Work out the finished part from the listing and answer in its coordinate system (mm). Face numbers are marked on the shaded views. A direction names the side the tool comes from. Round coordinates to 2 decimals unless told otherwise and drop trailing zeros. Loops run counter-clockwise (first coordinate to the right, second up) from the corner with the lowest first, then second, coordinate; pieces in that order, holes last. Notation, with made-up numbers: (-29, 50.25) - (-18, 50.25) arc R23 cw to (-18, 79.25) - close; hole circle Ø7 at (-3, 82.5). An arc over 180 degrees is marked (long way). Return JSON: item names as keys, results as strings.
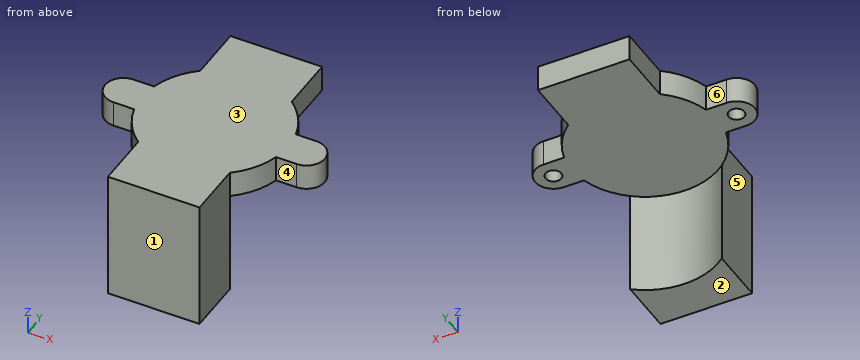
Autodesk Fusion 360 part; units mm, degrees
sketch "Sketch1" plane through (0, 0, 24.0553) normal (0, 0, 1) x (-1, 0, 0)
  line L0 (10.7499, 16.3506) -> (10.7499, 5.6583)
  line L1 (10.7499, 5.6583) -> (-6.7501, 5.6583)
  line L2 (-6.7501, 5.6583) -> (-6.7501, 16.3506)
  arc A0 (-11.5555, 23.7794) -> (-6.7501, 16.3506) centre (1.9999, 27.2794) ccw
  line L3 (-11.5555, 23.7794) -> (-15.5001, 23.7794)
  arc A1 (-15.5001, 30.7794) -> (-15.5001, 23.7794) centre (-15.5001, 27.2794) ccw
  line L4 (-15.5001, 30.7794) -> (-11.5555, 30.7794)
  arc A2 (-6.7501, 38.2081) -> (-11.5555, 30.7794) centre (1.9999, 27.2794) ccw
  line L5 (-6.7501, 38.2081) -> (-6.7501, 48.9005)
  line L6 (-6.7501, 48.9005) -> (10.7499, 48.9005)
  line L7 (10.7499, 48.9005) -> (10.7499, 38.2081)
  arc A3 (15.5554, 30.7794) -> (10.7499, 38.2081) centre (1.9999, 27.2794) ccw
  line L8 (15.5554, 30.7794) -> (19.4999, 30.7794)
  arc A4 (19.4999, 23.7794) -> (19.4999, 30.7794) centre (19.4999, 27.2794) ccw
  line L9 (19.4999, 23.7794) -> (15.5554, 23.7794)
  arc A5 (10.7499, 16.3506) -> (15.5554, 23.7794) centre (1.9999, 27.2794) ccw
  arc A6 (51.4999, 44.5294) -> (41.4999, 54.5294) centre (41.4999, 44.5294) ccw
  line L10 (41.4999, 54.5294) -> (-37.5001, 54.5294)
  arc A7 (-37.5001, 54.5294) -> (-47.5001, 44.5294) centre (-37.5001, 44.5294) ccw
  line L11 (-47.5001, 44.5294) -> (-47.5001, -34.4706)
  arc A8 (-47.5001, -34.4706) -> (-37.5001, -44.4706) centre (-37.5001, -34.4706) ccw
  line L12 (-37.5001, -44.4706) -> (41.4999, -44.4706)
  arc A9 (41.4999, -44.4706) -> (51.4999, -34.4706) centre (41.4999, -34.4706) ccw
  line L13 (51.4999, -34.4706) -> (51.4999, 44.5294)
  line L14 (42.9999, -37.9706) -> (-39.0001, -37.9706)
  line L15 (-39.0001, -37.9706) -> (-39.0001, 0.0294)
  line L16 (-39.0001, 0.0294) -> (42.9999, 0.0294)
  line L17 (42.9999, 0.0294) -> (42.9999, -37.9706)
  line L18 (10.7499, 48.9005) -> (10.7499, 38.2081)
  line L19 (-6.7501, 48.9005) -> (10.7499, 48.9005)
  line L20 (-6.7501, 38.2081) -> (-6.7501, 48.9005)
  arc A10 (-6.7501, 38.2081) -> (-11.5555, 30.7794) centre (1.9999, 27.2794) ccw
  arc A11 (15.5554, 30.7794) -> (10.7499, 38.2081) centre (1.9999, 27.2794) ccw
  line L21 (15.5554, 30.7794) -> (19.4999, 30.7794)
  arc A12 (19.4999, 23.7794) -> (19.4999, 30.7794) centre (19.4999, 27.2794) ccw
  line L22 (19.4999, 23.7794) -> (15.5554, 23.7794)
  arc A13 (15.5524, 23.7794) -> (15.5583, 30.7794) centre (1.9999, 27.2908) ccw
  line L23 (15.5524, 23.7794) -> (19.4999, 23.7794)
  arc A14 (19.4999, 23.7794) -> (19.4999, 30.7794) centre (19.4999, 27.2794) ccw
  line L24 (19.4999, 30.7794) -> (15.5583, 30.7794)
  circle A15 centre (19.4999, 27.2794) radius 2
  arc A16 (-11.5585, 30.7794) -> (-11.5526, 23.7794) centre (1.9999, 27.2908) ccw
  line L25 (-11.5585, 30.7794) -> (-15.5001, 30.7794)
  arc A17 (-15.5001, 30.7794) -> (-15.5001, 23.7794) centre (-15.5001, 27.2794) ccw
  line L26 (-15.5001, 23.7794) -> (-11.5526, 23.7794)
  circle A18 centre (-15.5001, 27.2794) radius 2
  line L27 (-6.7501, 5.6583) -> (-6.7501, 16.3506)
  line L28 (10.7499, 5.6583) -> (-6.7501, 5.6583)
  line L29 (10.7499, 16.3506) -> (10.7499, 5.6583)
  circle A19 centre (1.9999, 27.2908) radius 14
  arc A20 (-15.5001, 30.7794) -> (-15.5001, 23.7794) centre (-15.5001, 27.2794) ccw
  line L30 (-15.5001, 30.7794) -> (-11.5555, 30.7794)
  line L31 (-11.5555, 23.7794) -> (-15.5001, 23.7794)
  arc A21 (-11.5555, 23.7794) -> (-6.7501, 16.3506) centre (1.9999, 27.2794) ccw
  arc A22 (10.7499, 16.3506) -> (15.5554, 23.7794) centre (1.9999, 27.2794) ccw
  circle A23 centre (1.9999, 27.2908) radius 13
  circle A24 centre (19.4999, 27.2794) radius 1.5
  circle A25 centre (-15.5001, 27.2794) radius 1.5
extrude "Extrude2" add sketch "Sketch1" against normal blind 5 contours L0 L1 L2 A0 A5 L23 L26 L27 L28 L29 A19 A21 A22 | L8 A4 L9 L21 A12 L22 A13 L23 A14 L24 A19 | L4 A2 L5 L7 A3 L8 L18 L20 A10 A11 L21 A13 A16 A19 L30 | L3 A1 L4 A16 L25 A17 L26 A19 A20 L30 L31 | L7 A3 L8 L18 A11 L21 A19 | L4 A2 L5 L20 A10 A19 L30 | A23 makes body 1
extrude "Extrude1" add sketch "Sketch1" against normal blind 25 separate body contours L5 L6 L7 L18 L19 L20 A19 makes body 2
extrude "Extrude3" add sketch "Sketch1" against normal blind 4 separate body contours A15 | A18 makes body 3 at (-21.4974, -27.1797, 21.3887) makes body 4 at (13.5026, -27.1797, 21.3887)
sketch "Sketch2" plane through (0, 0, 24.0553) normal (0, 0, 1) x (-1, 0, 0)
  circle A0 centre (19.4999, 27.2794) radius 1.5
  circle A1 centre (19.4999, 27.2794) radius 1.5
extrude "Extrude4" add sketch "Sketch2" against normal blind 2 bodies 3
sketch "Sketch3" plane through (0, 0, 24.0553) normal (0, 0, 1) x (-1, 0, 0)
  circle A0 centre (-15.5001, 27.2794) radius 1.5
  circle A1 centre (-15.5001, 27.2794) radius 1.5
extrude "Extrude5" add sketch "Sketch3" against normal blind 2 bodies 4
extrude "Extrude6" add 1 faces at (13.7846, -26.6463, 20.0553) along direction (0, 0, -1) blind 1 on bodies 4 bodies 4 1
extrude "Extrude7" add 1 faces at (-18.7404, -28.9428, 20.0553) along direction (0, 0, -1) blind 1 on bodies 3 bodies 3 2 4
sketch "Sketch4" plane through (0, 0, 24.0553) normal (0, 0, 1) x (-1, 0, 0)
  line L0 (10.7499, 5.6583) -> (10.7499, 16.3506)
  arc A0 (10.7499, 16.3506) -> (15.5554, 23.7794) centre (1.9999, 27.2794) ccw
  line L1 (15.5554, 23.7794) -> (19.4999, 23.7794)
  arc A1 (19.4999, 23.7794) -> (19.4999, 30.7794) centre (19.4999, 27.2794) ccw
  line L2 (19.4999, 30.7794) -> (15.5554, 30.7794)
  arc A2 (15.5554, 30.7794) -> (10.7499, 38.2081) centre (1.9999, 27.2794) ccw
  line L3 (10.7499, 38.2081) -> (10.7499, 38.2196)
  arc A3 (10.7499, 38.2196) -> (-6.7501, 38.2196) centre (1.9999, 27.2908) ccw
  line L4 (-6.7501, 38.2196) -> (-6.7501, 38.2081)
  arc A4 (-6.7501, 38.2081) -> (-11.5555, 30.7794) centre (1.9999, 27.2794) ccw
  line L5 (-11.5555, 30.7794) -> (-15.5001, 30.7794)
  arc A5 (-15.5001, 30.7794) -> (-15.5001, 23.7794) centre (-15.5001, 27.2794) ccw
  line L6 (-15.5001, 23.7794) -> (-11.5555, 23.7794)
  arc A6 (-11.5555, 23.7794) -> (-6.7501, 16.3506) centre (1.9999, 27.2794) ccw
  line L7 (-6.7501, 16.3506) -> (-6.7501, 5.6583)
  line L8 (-6.7501, 5.6583) -> (10.7499, 5.6583)
  line L9 (10.7499, 48.9005) -> (-6.7501, 48.9005)
  line L10 (-6.7501, 48.9005) -> (-6.7501, 38.2196)
  arc A7 (10.7499, 38.2196) -> (-6.7501, 38.2196) centre (1.9999, 27.2908) ccw
  line L11 (10.7499, 38.2196) -> (10.7499, 48.9005)
  line L12 (10.7499, 38.2196) -> (10.7499, 48.9005)
  line L13 (-6.7501, 48.9005) -> (-6.7501, 38.2196)
  circle A8 centre (1.9999, 27.2908) radius 14
extrude "Extrude8" add sketch "Sketch4" against normal blind 25 contours A3 L9 L10 A7 L11 L12 L13 A8 bodies 2 3
1) Section A-A (z = 21) is taken. Give the vertices of the cut face in (x, y), and give its area (3 significant figures).
Verdict:
{"outline": "(-19.5, -30.78) - (-15.56, -30.78) arc R14 ccw to (-10.75, -38.22) - (-10.75, -48.9) - (6.75, -48.9) - (6.75, -38.22) arc R14 ccw to (11.56, -30.78) - (15.5, -30.78) arc R3.5 ccw to (15.5, -23.78) - (11.56, -23.78) arc R14 ccw to (6.75, -16.35) - (6.75, -5.66) - (-10.75, -5.66) - (-10.75, -16.35) arc R14 ccw to (-15.56, -23.78) - (-19.5, -23.78) arc R3.5 ccw to start; hole circle Ø3 at (-19.5, -27.28); hole circle Ø3 at (15.5, -27.28)", "area": "992 mm2"}
2) A tool of negligible diameter and unlimited length cuts with its end or side. For the marked faces 4, 5 and 6, from which of +Z, -Z, +X, -X, +Y, -Y can it reach the whole face along a straight path? Write none if from no direction.
Verdict:
{"face 4": "+Z, -Z, +X, -Y", "face 5": "+Z, -Z, -X, -Y", "face 6": "+Z, -Z, -X, +Y"}
3) Section C-C (x = -6.5) is taken. Give the vertices of the cut face in (y, z), and give its area (3 significant figures).
Verdict:
{"outline": "(-48.9, -0.94) - (-40.55, -0.94) - (-40.55, 19.06) - (-5.66, 19.06) - (-5.66, 24.06) - (-48.9, 24.06) - close", "area": "383 mm2"}
4) Flat-ended cylindrical pins translate along their axes: pin 1 (4 mm diameter, centred on y = -12.5, z = 22, fed in from +X); pin 2 (2 mm diameter, centred on x = 13.5, z = 21, fed in from +Y); pin 3 (4.5 mm diameter, centred on x = -16.5, z = 21.5, fed in from -Y); pin 4 (3 mm diameter, centred on x = -11.5, z = 18.5, fed in from +Y). Find the tip coordinate at first contact, or state that the pin passes through.
Verdict:
{"pin 1": "stops at x = 6.75", "pin 2": "stops at y = -23.78", "pin 3": "stops at y = -34.07", "pin 4": "stops at y = -5.66"}
5) Section B-B (y = -39.5) is taken. Give the vertices of the cut face in (x, z).
Verdict:
{"outline": "(-10.75, -0.94) - (-8.85, -0.94) - (-8.85, 19.06) - (4.85, 19.06) - (4.85, -0.94) - (6.75, -0.94) - (6.75, 24.06) - (-10.75, 24.06) - close"}
6) Determine the mould class of the marked faces 1, 2 and 3 for opening direction Z: pulls with the +Z half, pulls with the -Z half, needs draft (parallel to the pull), parting line crosses it, or undercut.
Verdict:
{"face 1": "needs draft", "face 2": "pulls with the -Z half", "face 3": "pulls with the +Z half"}
7) Find the intervals of material crossed by L1, parallel to Z at x = 3.5, y = -17; L2, parallel to X at y = -46, z = 7; L3, parallel to Y at x = -18.5, z = 20, in increasing order.
Verdict:
{"L1": "z = 19.06 to 24.06", "L2": "x = -10.75 to 6.75", "L3": "y = -30.78 to -28.4, -26.16 to -23.78"}
8) Section D-D (z = 17) is taken. Give the vertices of the cut face in (x, y).
Verdict:
{"outline": "(-10.75, -48.9) - (6.75, -48.9) - (6.75, -38.22) arc R14 cw to (-10.75, -38.22) - close"}
